Autodesk Inventor part; units mm, degrees
ref_plane "YZ Plane" through (0, 0, 0) normal (1, 0, 0) x (0, 1, 0)
ref_plane "XZ Plane" through (0, 0, 0) normal (0, 1, 0) x (-1, 0, 0)
ref_plane "XY Plane" through (0, 0, 0) normal (0, 0, 1) x (1, 0, 0)
sketch "Sketch1" plane through (0, 0, 0) normal (0, 1, 0) x (-1, 0, 0)
  line L0 (-1224.9972, -38) -> (-960.8978, -2044.0342)
  line L1 (-951.0627, -2080.7394) -> (232.1938, -1763.6868)
  line L2 (-955.895, -2082.0342) -> (274.105, -2082.0342) construction
  line L3 (227.191, -1725.6868) -> (5.0028, -38)
  line L4 (190.1691, -1735.6068) -> (-33.3251, -38)
  line L5 (-33.3251, -38) -> (-1186.6693, -38)
  line L6 (-1186.6693, -38) -> (-923.8759, -2034.1142)
  line L7 (-960.8978, -2044.0342) -> (-951.0627, -2080.7394)
  line L8 (-923.8759, -2034.1142) -> (190.1691, -1735.6068)
  line L9 (-1224.9972, -38) -> (-1224.9972, 0)
  line L10 (5.0028, -38) -> (5.0028, 0)
  line L11 (-1230, 0) -> (-1224.9972, 0) construction
  line L12 (5.0028, 0) -> (870, 0) construction
  line L13 (5.0028, 0) -> (-1224.9972, 0)
  line L14 (232.1938, -1763.6868) -> (237.0261, -1762.392)
  line L15 (227.191, -1725.6868) -> (237.0261, -1762.392)
  dimension "d1" = 2100
  dimension "d9" = 1230
  dimension "d10" = 15
  dimension "d12" = 38
extrude "Extrusion1" add sketch "Sketch1" along normal blind 114
sketch "Sketch2" plane through (0, 114, 0) normal (0, 1, 0) x (1, 0, 0)
  line L0 (33.3251, 38) -> (-190.1691, 1735.6068)
  line L1 (-227.191, 1725.6868) -> (-5.0028, 38)
  line L2 (1224.9972, 0) -> (1224.9972, 38)
  line L3 (960.8978, 2044.0342) -> (951.0627, 2080.7394)
  line L4 (-190.1691, 1735.6068) -> (-227.191, 1725.6868)
  line L5 (33.3251, 38) -> (-5.0028, 38)
  point P0 (0, 0)
extrude "Extrusion2" cut sketch "Sketch2" against normal blind 1
sketch "Sketch3" plane through (0, 114, 0) normal (0, 1, 0) x (1, 0, 0)
  line L0 (1224.9972, 0) -> (1224.9972, 38)
  line L1 (1224.9972, 38) -> (960.8978, 2044.0342)
  line L2 (960.8978, 2044.0342) -> (951.0627, 2080.7394)
  line L3 (951.0627, 2080.7394) -> (-237.0261, 1762.392)
  line L4 (-237.0261, 1762.392) -> (-227.191, 1725.6868)
  line L5 (-227.191, 1725.6868) -> (923.8759, 2034.1142)
  line L6 (923.8759, 2034.1142) -> (1186.6693, 38)
  line L7 (1186.6693, 38) -> (1224.9972, 38)
  line L8 (923.8759, 2034.1142) -> (960.8978, 2044.0342)
  point P0 (0, 0)
extrude "Extrusion3" cut sketch "Sketch3" against normal blind 1 contours L7 L6 L8 L1
properties part number "H7jp.E_UfaA-panelEframe" material "Wood (Cherry)"
Here's how the part is built. I have some questions about the finished solid (model axes, mm). Coordinates: 2 decimals unless noted, no trailing zeros. Order: outer loops, then holes, each group sorted by start corner. A loop starts at its lowest first (then second) coordinate and runs counter-clockwise, first axis right, second up.
1) I need wall thicknesses on line 1 (Z direction, x = 510, y = 100); line 2 (Z direction, x = 160, y = 15.5); line 3 (X direction, y = 56.5, z = -822.5). Which ranges of each line are inside material? Lowest first, please.
2) Imagine slicing it at B-B on x = 430.5. List the corners of the cut face in (y, z) for me.
3) Will these pins go through, and if not, where does the flat tip stop? pin 1 (5 mm diameter, centred on y = 55, z = -1181, fed in from +X); pin 2 (1 mm diameter, centred on y = 79, z = -1454, fed in from +X); pin 3 (4 mm diameter, centred on y = 75.5, z = -1743, fed in from -X).
4) Imagine slicing it at C-C on z = -128.5. List the corners of the cut face in (x, y) for me, and give its area (3 significant figures).
5) Imagine slicing it at A-A on y = 86.5. List the corners of the cut face in (x, z) for me, and give its area (3 significant figures).
6) We'd pull the mould along Z, two halves only. Please class faces 1 (the face through (1093, 0, -804)), 2 (the face through (-79.986, 55.709, -898.687)), 3 (the face through (1094.796, 55.709, -1026.975)), 4 (the face through (1057.112, 55.709, -1022.084)): +Z half, -Z half, draft (parallel to the pull), parting line (faces both ways), or undercut.
Response values:
1. line 1: z = -1962.56 to -1923.22, -38 to 0
1. line 2: z = -1868.77 to -1829.43, -38 to 0
1. line 3: x = -108.28 to -69.96, 1083.39 to 1121.72
2. outline: (0, -1941.26) - (114, -1941.26) - (114, -1901.91) - (0, -1901.91) - close; (0, -38) - (114, -38) - (114, 0) - (0, 0) - close
3. pin 1: stops at x = 1074.85
3. pin 2: stops at x = 1038.64
3. pin 3: stops at x = -232.37
4. outline: (-16.92, 0) - (21.41, 0) - (21.41, 113) - (-16.92, 113) - close; (1174.75, 0) - (1213.08, 0) - (1213.08, 113) - (1174.75, 113) - close
4. area: 8,660 mm2
5. outline: (-237.03, -1762.39) - (-232.19, -1763.69) - (951.06, -2080.74) - (960.9, -2044.03) - (1225, -38) - (1225, 0) - (-5, 0) - (-5, -38) - (-227.19, -1725.69) - close; hole (-190.17, -1735.61) - (923.88, -2034.11) - (1186.67, -38) - (33.33, -38) - close
5. area: 235,000 mm2
6. face 1: draft
6. face 2: undercut
6. face 3: -Z half
6. face 4: undercut
